Part model, mm, in its own coordinate system. Face numbers are marked on the shaded views. A direction names the side the tool comes from. Coordinates: 2 decimals unless noted, no trailing zeros. Order: outer loops, then holes, each group sorted by start corner. A loop starts at its lowest first (then second) coordinate and runs counter-clockwise, first axis right, second up.
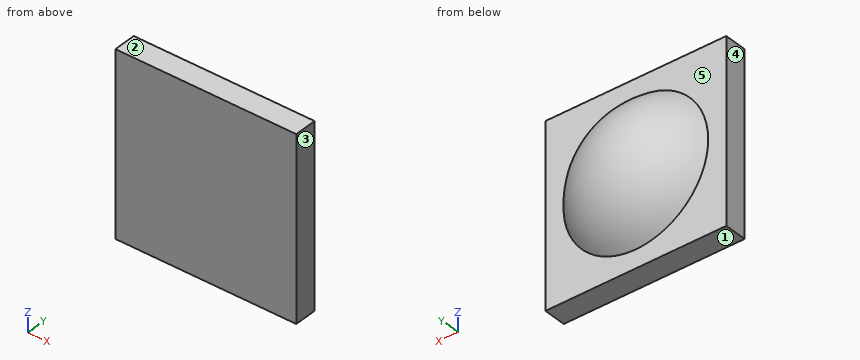
from build123d import *

# Parameters (mm, degrees)
SKETCH1_W           = 50.8
SKETCH1_H           = 50.8
BOSS_EXTRUDE1_DEPTH = 6.35


with BuildPart() as part:
    # Sketch1 → Boss-Extrude1 (new body)
    with BuildSketch(Plane(origin=(0, 0, 0), x_dir=(1, 0, 0), z_dir=(0, 1, 0))):
        Rectangle(SKETCH1_W, SKETCH1_H)
    extrude(amount=BOSS_EXTRUDE1_DEPTH)

    # Sketch2 → Revolve1 (revolve)
    with BuildSketch(Plane.XY):
        with BuildLine():
            Line((0, 6.35), (-20.32, 6.35))
            ThreePointArc((-20.32, 6.35), (-11.359225326, 13.828450651), (0, 16.51))
            Line((0, 16.51), (0, 6.35))
        make_face()
    revolve(axis=Axis((0, 16.51, 0), (0, -1, 0)))


solid = part.part
Q1. Cut at D-D on y = 7.5. Write the cut outline in (x, z), and give its area (3 significant figures).
Results list:
outline: circle Ø38.81 at (0, 0)
area: 1,180 mm2
Q2. Which spindle directions (+Z, -Z, +X, -X, +Y, -Y) get a long thin tool onto all of the face, cutting with end or side? Do the marked faces 4 and 5. Say none if no direction does.
Results list:
face 4: +Z, -Z, -X, +Y, -Y
face 5: +Y
Q3. Cut at A-A on x = -8.5. Write the cut outline in (y, z).
Results list:
outline: (0, -25.4) - (6.35, -25.4) - (6.35, -18.46) arc R23.94 ccw to (6.35, 18.46) - (6.35, 25.4) - (0, 25.4) - close
Q4. Mould opens along Z. For the marked faces 1, 2 and 3 say: pulls with the +Z half, pulls with the -Z half, needs draft (parallel to the pull), parting line crosses it, or undercut.
Results list:
face 1: pulls with the -Z half
face 2: pulls with the +Z half
face 3: needs draft
Q5. Cut at B-B on z = -16. Write the cut outline in (x, y).
Results list:
outline: (-25.4, 0) - (25.4, 0) - (25.4, 6.35) - (12.53, 6.35) arc R19.73 ccw to (-12.53, 6.35) - (-25.4, 6.35) - close
Q6. Cut at C-C on y = 13.25. Write the cut outline in (x, z), and give its area (3 significant figures).
Results list:
outline: circle Ø24.9 at (0, 0)
area: 487 mm2
Q7. Wall check: line 1 along Y through (x, z) = (21, -13.5); line 2 along Z through (x, y) = (-8, 11.75); line 3 along Y through (x, z) = (6, 18). Give the ranges that are in metal, low to high.
Results list:
line 1: y = 0 to 6.35
line 2: z = -12.46 to 12.46
line 3: y = 0 to 8
Q8. Pin check, flat tips, straight feed: pin 1 Ø4 at (x, z) = (-7.5, 15.5) entering from +Y; pin 2 Ø3 at (y, z) = (9.5, -4) entering from -X; pin 3 Ø4 at (y, z) = (9, 3.5) entering from +X. Stop position of each tip, or through.
Results list:
pin 1: stops at y = 11.45
pin 2: stops at x = -18.58
pin 3: stops at x = 19.54
